Build history of the part. All positions in model axes, mm. A direction names the side the tool comes from. Round coordinates to 2 decimals unless told otherwise and drop trailing zeros. Write each loop counter-clockwise with the first axis right and the second up, starting at its lowest first coordinate (ties: lowest second). Pieces come first, ordered by that corner, then holes.
Item 1: Mould opens along Z. For faces 5 (the cylindrical face through (23.976, 28.353, 4.834)), 6 (the cylindrical face through (148.784, 12.451, -72.488)), 7 (the flat face through (146, 44.45, -64)), 8 (the flat face through (34.3, 28.4, 13.1)) say: +Z half, -Z half, draft (parallel to the pull), parting line (faces both ways), or undercut.
Item 2: Drop flat-ended pins along their axis: pin 1 Ø5 at (x, z) = (129, -62.5) entering from +Y; pin 2 Ø2 at (x, z) = (121.28, -63.82) entering from -Y; pin 3 Ø5 at (y, z) = (30, -65) entering from -X; pin 4 Ø1 at (x, y) = (26, 12.5) entering from +Z. Give the stop position or say it passes through.
Item 3: Band-saw the part on D-D, the plane x = 131. Write the cut outline in (y, z), then the cut area to 3 significant figures.
Item 4: Band-saw the part on B-B, the plane z = -19.05. Write the cut outline in (x, y) (3 decimals).
Item 5: Band-saw the part on A-A, the plane y = 33. Count the separate pieces of the cut face and the enclosed holes in it, then the cut area to 3 significant figures.
Item 6: Wall check: probe 1 along Y at (x, z) = (116, -53.5); probe 2 along Z at (x, y) = (27, 3.5); probe 3 along Z at (x, y) = (11, 7.5). Give the ranges that are in metal, low to high.
Item 7: 3-axis set-ups, long thin cutter, end or side, ignore diameter. For faces 1 (the flat face through (11.94, 28.35, 0.24)), 2 (the flat face through (23, 44.45, 8)), 3 (the flat face through (34.28, 28.35, -140.78)), 4 (the flat face through (145.15, 28.35, -76.71)): which of +Z, -Z, +X, -X, +Y, -Y reach the whole face in a straight line?
```python
from build123d import *

# Parameters (mm, degrees)
SKETCH1_W           = 127.635
SKETCH1_H           = 127.635
MAIN_PLATE_DEPTH    = 12.7
SKETCH9_R           = 85.725
BOSS_EXTRUDE1_DEPTH = 12.7
SKETCH10_R          = 95.25
SKETCH10_R_2        = 85.4075
CUT_EXTRUDE1_DEPTH  = 167.64
SKETCH18_R          = 85.4075
SKETCH18_R_2        = 79.375
BOSS_EXTRUDE2_DEPTH = 38.1
SKETCH21_R          = 15.875
SKETCH21_R_2        = 1.778
CO2_MOUNTS_DEPTH    = 13.7
SKETCH22_R          = 5.08
CUT_EXTRUDE5_DEPTH  = 13.7
SKETCH23_R          = 79.375
CUT_EXTRUDE6_DEPTH  = 111.600000066


with BuildPart() as part:
    # Sketch1 → Main Plate (new body)
    with BuildSketch(Plane(origin=(0, 0, 0), x_dir=(1, 0, 0), z_dir=(0, 1, 0))):
        with Locations((63.8175, 63.8175)):
            Rectangle(SKETCH1_W, SKETCH1_H)
    extrude(amount=MAIN_PLATE_DEPTH)

    # Sketch9 → Boss-Extrude1 (add)
    with BuildSketch(Plane(origin=(0, 12.7, 0), x_dir=(1, 0, 0), z_dir=(0, 1, 0))):
        with Locations((63.8175, 63.8175)):
            Circle(SKETCH9_R)
    extrude(amount=-BOSS_EXTRUDE1_DEPTH)

    # Sketch10 → Cut-Extrude1 (cut)
    with BuildSketch(Plane(origin=(0, 12.7, 0), x_dir=(1, 0, 0), z_dir=(0, 1, 0))):
        with Locations((63.8175, 63.8175)):
            Circle(SKETCH10_R)
        with Locations((63.8175, 63.8175)):
            Circle(SKETCH10_R_2, mode=Mode.SUBTRACT)
    extrude(amount=-CUT_EXTRUDE1_DEPTH, mode=Mode.SUBTRACT)

    # Sketch18 → Boss-Extrude2 (add)
    with BuildSketch(Plane(origin=(0, 6.35, 0), x_dir=(1, 0, 0), z_dir=(0, 1, 0))):
        with Locations((63.8175, 63.8175)):
            Circle(SKETCH18_R)
        with Locations((63.8175, 63.8175)):
            Circle(SKETCH18_R_2, mode=Mode.SUBTRACT)
    extrude(amount=BOSS_EXTRUDE2_DEPTH)

    # Sketch21 → CO2 Mounts (cut, through all)
    with BuildSketch(Plane(origin=(0, 12.7, 0), x_dir=(1, 0, 0), z_dir=(0, 1, 0))):
        with Locations((102.235, 63.8175)):
            Circle(SKETCH21_R)
        with Locations((102.235, 82.8675)):
            Circle(SKETCH21_R_2)
        with Locations((25.4, 63.8175)):
            Circle(SKETCH21_R)
        with Locations((121.285, 63.8175)):
            Circle(SKETCH21_R_2)
        with Locations((102.235, 44.7675)):
            Circle(SKETCH21_R_2)
        with Locations((83.185, 63.8175)):
            Circle(SKETCH21_R_2)
        with Locations((25.4, 82.8675)):
            Circle(SKETCH21_R_2)
        with Locations((6.35, 63.8175)):
            Circle(SKETCH21_R_2)
        with Locations((25.4, 44.7675)):
            Circle(SKETCH21_R_2)
        with Locations((44.45, 63.8175)):
            Circle(SKETCH21_R_2)
    extrude(amount=-CO2_MOUNTS_DEPTH, mode=Mode.SUBTRACT)

    # Sketch22 → Cut-Extrude5 (cut, through all)
    with BuildSketch(Plane(origin=(0, 12.7, 0), x_dir=(1, 0, 0), z_dir=(0, 1, 0))):
        with Locations((46.355, 108.585)):
            Circle(SKETCH22_R)
        with Locations((81.28, 108.585)):
            Circle(SKETCH22_R)
        with Locations((81.28, 19.05)):
            Circle(SKETCH22_R)
        with Locations((46.355, 19.05)):
            Circle(SKETCH22_R)
    extrude(amount=-CUT_EXTRUDE5_DEPTH, mode=Mode.SUBTRACT)

    # Sketch23 → Cut-Extrude6 (cut)
    with BuildSketch(Plane(origin=(0, 12.7, 0), x_dir=(1, 0, 0), z_dir=(0, 1, 0))):
        with Locations((63.8175, 63.8175)):
            Circle(SKETCH23_R)
        with BuildLine():
            Line((13.678739997, 125.352005526), (7.552270878, 134.237860218))
            Line((7.552270878, 134.237860218), (-19.267108419, 125.320629884))
            Line((-19.267108419, 125.320629884), (-48.79695837, 60.397770071))
            Line((-48.79695837, 60.397770071), (-9.884344094, 7.052469015))
            Line((-9.884344094, 7.052469015), (6.959175986, -7.46308736))
            Line((6.959175986, -7.46308736), (13.678739997, 2.282994474))
            ThreePointArc((13.678739997, 2.282994474), (-15.5575, 63.8175), (13.678739997, 125.352005526))
        make_face()
        with BuildLine():
            Line((142.177324996, 76.471687114), (152.935935453, 77.334437661))
            Line((152.935935453, 77.334437661), (158.623077101, 105.019316613))
            Line((158.623077101, 105.019316613), (117.163156193, 163.054346747))
            Line((117.163156193, 163.054346747), (51.508463168, 156.027684783))
            Line((51.508463168, 156.027684783), (30.515862556, 148.698546693))
            Line((30.515862556, 148.698546693), (35.596435007, 138.00619264))
            ThreePointArc((35.596435007, 138.00619264), (103.505, 132.558266425), (142.177324996, 76.471687114))
        make_face()
        with BuildLine():
            Line((35.596435007, -10.37119264), (30.964293669, -20.119797879))
            Line((30.964293669, -20.119797879), (52.096531318, -38.887446496))
            Line((52.096531318, -38.887446496), (123.086302178, -31.999616818))
            Line((123.086302178, -31.999616818), (149.828380926, 28.372346201))
            Line((149.828380926, 28.372346201), (153.977461458, 50.217040667))
            Line((153.977461458, 50.217040667), (142.177324996, 51.163312886))
            ThreePointArc((142.177324996, 51.163312886), (103.505, -4.923266425), (35.596435007, -10.37119264))
        make_face()
    extrude(amount=CUT_EXTRUDE6_DEPTH, mode=Mode.SUBTRACT)


solid = part.part
```
Results:
1. face 5: undercut
1. face 6: parting line
1. face 7: draft
1. face 8: +Z half
2. pin 1: stops at y = 12.7
2. pin 2: passes through
2. pin 3: stops at x = 143.11
2. pin 4: stops at z = 13.01
3. outline: (0, -116.55) - (12.7, -116.55) - (12.7, -11.08) - (0, -11.08) - close
3. area: 1,340 mm2
4. outline: (-8.917, 0) - (41.275, 0) - (41.275, 12.7) - (-8.917, 12.7) - close; (51.435, 0) - (76.2, 0) - (76.2, 12.7) - (51.435, 12.7) - close; (86.36, 0) - (136.552, 0) - (136.552, 12.7) - (86.36, 12.7) - close
5. separate pieces: 3
5. enclosed holes: 0
5. area: 469 mm2
6. probe 1: y = 0 to 12.7
6. probe 2: z = -140.88 to -83.64, -82.09 to -79.61, -48.02 to -45.54, -43.99 to 13.25
6. probe 3: z = -130.93 to -70.5, -57.14 to 3.3
7. face 1: -X, +Y
7. face 2: +Z, -Z, +X, -X, +Y
7. face 3: -Z, +X, +Y
7. face 4: -Z, -X, +Y
